CAD build for the part. Positions are in the model's coordinates, mm. Face numbers are marked on the shaded views. A direction names the side the tool comes from. Give positions to 0.01 mm unless a question says otherwise; leave off trailing zeros. Loops run counter-clockwise (first coordinate to the right, second up) from the corner with the lowest first, then second, coordinate; pieces in that order, holes last.
```python
from build123d import *

# Parameters (mm, degrees)
F1_DEPTH = 17.272
F2_DEPTH = 19.812
F3_R     = 3.483258


with BuildPart() as f1:
    # F0 (on Top) → F1 (new body, symmetric)
    with BuildSketch(Plane.XY):
        Polygon((0, 18.248798), (-8.939255, 7.643078), (-22.423375, 0), (-6.818111, -9.410581), (0, -20.386325), (8.939255, -7.643078), (25.605388, 0), (6.818111, 9.410581), align=None)
        Polygon((-16.059943, 0), (-6.818111, 5.689826), (0, 15.521614), (6.818111, 5.689826), (18.787423, 0), (6.818111, -5.689826), (0, -14.780444), (-6.818111, -5.689826), align=None, mode=Mode.SUBTRACT)
    extrude(amount=F1_DEPTH, both=True)

    # F0 (on Top) → F2 (join)
    with BuildSketch(Plane.XY):
        Polygon((0, 15.521614), (-6.818111, 5.689826), (-16.059943, 0), (-6.818111, -5.689826), (0, -14.780444), (6.818111, -5.689826), (18.787423, 0), (6.818111, 5.689826), align=None)
    extrude(amount=-F2_DEPTH)

    # F3
    f3_edges = [f1.edges().sort_by_distance(p)[0] for p in [
        (0, -20.386325, 0),
        (-22.423375, 0, 0),
        (0, 18.248798, 0),
        (25.605388, 0, 0),
    ]]
    fillet(f3_edges, radius=F3_R)


solid = f1.part
```
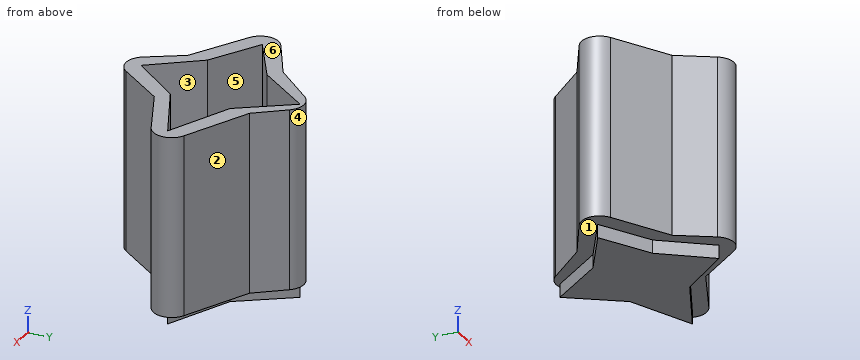
1. Saw through at A-A, the plane z = 10.5. List the corners of the cut face in (x, y), and give its area (3 significant figures).
Responses:
outline: (-17.32, -3.08) - (-6.82, -9.41) - (-2.78, -15.91) arc R3.48 ccw to (3.03, -16.07) - (8.94, -7.64) - (19, -3.03) arc R3.48 ccw to (19.11, 3.25) - (6.82, 9.41) - (2.64, 14.83) arc R3.48 ccw to (-2.78, 14.95) - (-8.94, 7.64) - (-17.24, 2.94) arc R3.48 ccw to start; hole (-16.06, 0) - (-6.82, -5.69) - (0, -14.78) - (6.82, -5.69) - (18.79, 0) - (6.82, 5.69) - (0, 15.52) - (-6.82, 5.69) - close
area: 279 mm2
2. Drop flat-ended pins along their axis: pin 1 (8 mm diameter, centred on x = 5.5, y = 11.5, fed in from -Z); pin 2 (1 mm diameter, centred on x = -7.5, z = 7.5, fed in from +Y); pin 3 (6 mm diameter, centred on x = 3, z = -5, fed in from +Y); pin 4 (5 mm diameter, centred on x = 16.5, z = 5.5, fed in from +Y). Give the stop position or say it passes through.
Responses:
pin 1: stops at z = -19.81
pin 2: stops at y = 9.94
pin 3: stops at y = 16.18
pin 4: stops at y = 5.81
3. Saw through at C-C, the plane z = -6. List the corners of the cut face in (x, y), and give its area (3 significant figures).
Responses:
outline: (-17.32, -3.08) - (-6.82, -9.41) - (-2.78, -15.91) arc R3.48 ccw to (3.03, -16.07) - (8.94, -7.64) - (19, -3.03) arc R3.48 ccw to (19.11, 3.25) - (6.82, 9.41) - (2.64, 14.83) arc R3.48 ccw to (-2.78, 14.95) - (-8.94, 7.64) - (-17.24, 2.94) arc R3.48 ccw to start
area: 684 mm2
4. Tool access for the marked faces 1, 2 and 3: list every direction of +Z, -Z, +X, -X, +Y, -Y with a clear straight run to the whole face (end or side of a thin tool).
Responses:
face 1: -Z
face 2: +Z, -Z, +X, +Y
face 3: +Z
5. Probe line 1 along Z through (x, y) = (-8, 8); line 2 along X through (y, z) = (-10, 16); line 3 along X through (y, z) = (-6, 6). List the from-to ranges inside material, lowest first.
Responses:
line 1: z = -17.27 to 17.27
line 2: x = -6.45 to -3.59, 3.59 to 7.29
line 3: x = -12.47 to -6.59, 6.59 to 12.52
6. Saw through at B-B, the plane y = 13.5. List the corners of the cut face in (x, z).
Responses:
outline: (-4, -17.27) - (-1.4, -17.27) - (-1.4, -19.81) - (1.4, -19.81) - (1.4, -17.27) - (3.66, -17.27) - (3.66, 17.27) - (1.4, 17.27) - (1.4, 0) - (-1.4, 0) - (-1.4, 17.27) - (-4, 17.27) - close
7. Pull direction Y, two halves, no side cores. Call the marked faces 4, 5 and 6: released by +Y, released by -Y, zero draft, split by the parting line, or undercut.
Responses:
face 4: released by +Y
face 5: undercut
face 6: zero draft
